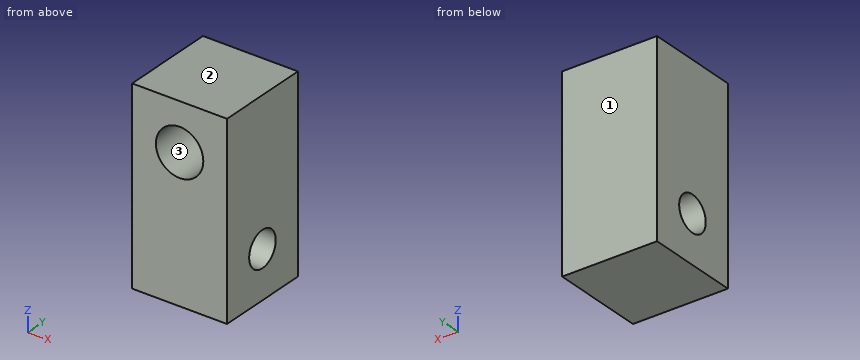
from build123d import *

# Parameters (mm, degrees)
F0_W     = 25.4
F0_H     = 50.8
F1_DEPTH = 25.4
F2_R     = 6.35
F3_DEPTH = 19.05
F4_R     = 4.7625
F5_DEPTH = 25.4


with BuildPart() as f1:
    # F0 (on Front) → F1 (new body)
    with BuildSketch(Plane.XZ):
        with Locations((-12.958675, -15.683598)):
            Rectangle(F0_W, F0_H)
    extrude(amount=F1_DEPTH)

    # F2 (on face) → F3 (cut)
    with BuildSketch(Plane.XZ.offset(25.4)):
        with Locations((-12.958675, -2.983598)):
            Circle(F2_R)
    extrude(amount=-F3_DEPTH, mode=Mode.SUBTRACT)

    # F4 (on face) → F5 (cut)
    with BuildSketch(Plane.YZ.offset(-0.258675)):
        with Locations((-12.7, -28.383598)):
            Circle(F4_R)
    extrude(amount=-F5_DEPTH, mode=Mode.SUBTRACT)


solid = f1.part
Model file for the job. Use its own axes, mm. Face numbers are marked on the shaded views. Round coordinates to 2 decimals unless told otherwise and drop trailing zeros. Loops run counter-clockwise (first coordinate to the right, second up) from the corner with the lowest first, then second, coordinate; pieces in that order, holes last. Notation, with made-up numbers: (6.25, 8.5) -> (33.25, 8.5) arc R8 cw to (33.25, 23.5) -> close; hole circle Ø1 at (-36.75, 15.5). An arc over 180 degrees is marked (long way). Answer as CSV lines item,"result". Start each with the question number.
1) Slice it at A-A (y = -11.5). List the corners of the cut face in (x, z), plus the area to 3 significant figures.
2) Mould opens along Z. For the marked faces 1, 2 and 3 say: +Z half, -Z half, draft (parallel to the pull), parting line (faces both ways), or undercut.
3) Slice it at C-C (y = -8.75). List the corners of the cut face in (x, z), plus the area to 3 significant figures.
4) Slice it at D-D (x = -1.75). List the corners of the cut face in (y, z) (1 decimal), plus the area to 3 significant figures.
5) Probe line 1 along Z through (x, y) = (-8.75, -12.7); line 2 along Z through (x, y) = (-9.5, -15); line 3 along Y through (x, z) = (-8.5, -24). List the from-to ranges inside material, lowest first.
6) Pin check, flat tip, straight feed: P1, Ø4, axis at x = -11.5, z = -5, coming from the -Y side. Stop position of the tip, or through.
Filled in:
1,outline,"(-25.66, -41.08) -> (-0.26, -41.08) -> (-0.26, -32.99) -> (-25.66, -32.99) -> close; (-25.66, -23.77) -> (-0.26, -23.77) -> (-0.26, 9.72) -> (-25.66, 9.72) -> close; hole circle Ø12.7 at (-12.96, -2.98)"
1,area,"930 mm2"
2,face 1,"draft"
2,face 2,"+Z half"
2,face 3,"undercut"
3,outline,"(-25.66, -41.08) -> (-0.26, -41.08) -> (-0.26, -31.04) -> (-25.66, -31.04) -> close; (-25.66, -25.72) -> (-0.26, -25.72) -> (-0.26, 9.72) -> (-25.66, 9.72) -> close; hole circle Ø12.7 at (-12.96, -2.98)"
3,area,"1,030 mm2"
4,outline,"(-25.4, -41.1) -> (0, -41.1) -> (0, 9.7) -> (-25.4, 9.7) -> close; hole circle Ø9.5 at (-12.7, -28.4)"
4,area,"1,220 mm2"
5,line 1,"z = -41.08 to -33.15, -23.62 to -7.74, 1.77 to 9.72"
5,line 2,"z = -41.08 to -32.55, -24.21 to -8.31, 2.34 to 9.72"
5,line 3,"y = -25.4 to -14.56, -10.84 to 0"
6,P1,"stops at y = -6.35"
